Work out the finished part from the listing and answer in its coordinate system (mm). A direction names the side the tool comes from. Round coordinates to 2 decimals unless told otherwise and drop trailing zeros. Loops run counter-clockwise (first coordinate to the right, second up) from the corner with the lowest first, then second, coordinate; pieces in that order, holes last.
from build123d import *

# Parameters (mm, degrees)
BOSS_EXTRUDE1_DEPTH      = 6.5
BOSS_EXTRUDE1_DEPTH_BACK = 6.5
SKETCH1_R                = 30
SKETCH1_R_2              = 10.5
SKETCH1_R_3              = 2.5
SKETCH2_R                = 14.35
CUT_EXTRUDE1_DEPTH       = 7.9375
CUT_EXTRUDE3_START       = -6.5
SKETCH3_R                = 4.5
CUT_EXTRUDE3_DEPTH       = 6
CUT_EXTRUDE4_START       = 30
SKETCH4_R                = 2.1
CUT_EXTRUDE4_DEPTH       = 15


with BuildPart() as part:
    # Sketch1 → Boss-Extrude1 (new, two sides: drawn at the far end of the back side and taken through both)
    with BuildSketch(Plane(origin=(0, 0, 0), x_dir=(1, 0, 0), z_dir=(0, 1, 0)).offset(-BOSS_EXTRUDE1_DEPTH_BACK)):
        with Locations(Location((0, 0, 0), (0, 0, 270))):
            Circle(SKETCH1_R)
        with Locations(Location((0, 0, 0), (0, 0, 270))):
            Circle(SKETCH1_R_2, mode=Mode.SUBTRACT)
        with Locations(Location((17.67766953, 17.67766953, 0), (0, 0, 270))):
            Circle(SKETCH1_R_3, mode=Mode.SUBTRACT)
        with Locations(Location((17.67766953, -17.67766953, 0), (0, 0, 270))):
            Circle(SKETCH1_R_3, mode=Mode.SUBTRACT)
        with Locations(Location((-17.67766953, -17.67766953, 0), (0, 0, 270))):
            Circle(SKETCH1_R_3, mode=Mode.SUBTRACT)
        with Locations(Location((-17.67766953, 17.67766953, 0), (0, 0, 270))):
            Circle(SKETCH1_R_3, mode=Mode.SUBTRACT)
    extrude(amount=BOSS_EXTRUDE1_DEPTH + BOSS_EXTRUDE1_DEPTH_BACK)

    # Sketch2 → Cut-Extrude1 (cut)
    with BuildSketch(Plane(origin=(0, 0, 0), x_dir=(1, 0, 0), z_dir=(0, 1, 0))):
        with Locations(Location((0, 0, 0), (0, 0, 270))):
            Circle(SKETCH2_R)
    extrude(amount=CUT_EXTRUDE1_DEPTH, mode=Mode.SUBTRACT)

    # Sketch3 → Cut-Extrude3 (cut)
    with BuildSketch(Plane(origin=(0, 0, 0), x_dir=(1, 0, 0), z_dir=(0, 1, 0)).offset(CUT_EXTRUDE3_START)):
        with Locations(Location((17.67766953, 17.67766953, 0), (0, 0, 270))):
            Circle(SKETCH3_R)
        with Locations(Location((17.67766953, -17.67766953, 0), (0, 0, 270))):
            Circle(SKETCH3_R)
        with Locations(Location((-17.67766953, -17.67766953, 0), (0, 0, 270))):
            Circle(SKETCH3_R)
        with Locations(Location((-17.67766953, 17.67766953, 0), (0, 0, 270))):
            Circle(SKETCH3_R)
    extrude(amount=CUT_EXTRUDE3_DEPTH, mode=Mode.SUBTRACT)

    # Sketch4 → Cut-Extrude4 (cut)
    with BuildSketch(Plane.XY.offset(CUT_EXTRUDE4_START)):
        Circle(SKETCH4_R)
    extrude(amount=-CUT_EXTRUDE4_DEPTH, mode=Mode.SUBTRACT)


solid = part.part
Item 1: Straight lines are drawn through the part: line 1 (Z direction, x = 19, y = 0); line 2 (X direction, y = 3.5, z = 19.5); line 3 (X direction, y = 5.25, z = 16). For each, find the intervals that lie inside material, in ascending order.
Item 2: For faces 1 (the face through (-20, -0.5, 20)), 2 (the face through (-11, 0, 1)), 3 (the face through (0, 0, 15)), 4 (the face through (-13, -6.5, 0)), 5 (the face through (19.37, 2.95, -19.52)), determine the directions among +Z, -Z, +X, -X, +Y, -Y from which every point of the face is accessible in a straight line to the end or side of a thin tool.
Item 3: Section A-A, the plane x = 0 is taken. Give the vertices of the cut face in (y, z), plus the area to 3 significant figures.
Item 4: Determine the mould class of faces 6 (the face through (22.14, -3.54, -18.26)), 7 (the face through (7, 6.5, 13)), 8 (the face through (1.32, -0.09, -29.97)), 9 (the face through (22.14, -3.54, 17.09)) for opening direction X: pulls with the +X half, pulls with the -X half, needs draft (parallel to the pull), parting line crosses it, or undercut.
Item 5: Section B-B, the plane z = 0 is taken. Give the vertices of the cut face in (x, y).
Item 6: Each of these flat-tipped pins is pushed along its axis until it touches: P1, Ø1.5, axis at y = -4, z = -2, coming from the +X side; P2, Ø1.5, axis at y = 3.5, z = 10, coming from the +X side; P3, Ø4, axis at x = -19.5, y = -4, coming from the +Z side. Where does it stop, or does it pass through?
Item 7: Section C-C, the plane x = -19 is taken. Give the vertices of the cut face in (y, z).
Item 8: Section D-D, the plane y = 5.5 is taken. Give the vertices of the cut face in (x, z), plus the area to 3 significant figures.
Answer below:
1. line 1: z = -23.22 to -19.8, -15.56 to 15.56, 19.8 to 23.22
1. line 2: x = -22.8 to -19.39, -15.97 to 15.97, 19.39 to 22.8
1. line 3: x = -25.38 to -19.53, -15.82 to 15.82, 19.53 to 25.38
2. face 1: -Y
2. face 2: +Y
2. face 3: +Z
2. face 4: +Z, -Z, +X, -X, -Y
2. face 5: +Y, -Y
3. outline: (-6.5, -30) - (6.5, -30) - (6.5, -14.35) - (0, -14.35) - (0, -10.5) - (-6.5, -10.5) - close; (-6.5, 10.5) - (0, 10.5) - (0, 14.35) - (6.5, 14.35) - (6.5, 30) - (2.1, 30) - (2.1, 15) - (-2.1, 15) - (-2.1, 30) - (-6.5, 30) - close
3. area: 394 mm2
4. face 6: undercut
4. face 7: needs draft
4. face 8: parting line crosses it
4. face 9: undercut
5. outline: (-30, -6.5) - (-10.5, -6.5) - (-10.5, 0) - (-14.35, 0) - (-14.35, 6.5) - (-30, 6.5) - close; (10.5, -6.5) - (30, -6.5) - (30, 6.5) - (14.35, 6.5) - (14.35, 0) - (10.5, 0) - close
6. P1: stops at x = 29.97
6. P2: stops at x = 28.54
6. P3: stops at z = 24.37
7. outline: (-6.5, -23.22) - (6.5, -23.22) - (6.5, -19.8) - (-0.5, -19.8) - (-0.5, -21.98) - (-6.5, -21.98) - close; (-6.5, -13.38) - (-0.5, -13.38) - (-0.5, -15.56) - (6.5, -15.56) - (6.5, 15.56) - (-0.5, 15.56) - (-0.5, 13.38) - (-6.5, 13.38) - close; (-6.5, 21.98) - (-0.5, 21.98) - (-0.5, 19.8) - (6.5, 19.8) - (6.5, 23.22) - (-6.5, 23.22) - close
8. outline: circle Ø60 at (0, 0); hole circle Ø5 at (-17.68, -17.68); hole circle Ø5 at (-17.68, 17.68); hole circle Ø28.7 at (0, 0); hole circle Ø5 at (17.68, -17.68); hole circle Ø5 at (17.68, 17.68)
8. area: 2,100 mm2
